Source: CAD feature listing. Evaluate the final solid. Frame: model axes, mm. Round coordinates to 2 decimals unless told otherwise and drop trailing zeros. Loops run counter-clockwise (first coordinate to the right, second up) from the corner with the lowest first, then second, coordinate; pieces in that order, holes last.
Item 1: Section query D-D on z = 0.9. Return loops of the section in (x, y).
Item 2: Ray query, L1, parallel to X at y = 4, z = 1; L2, parallel to X at y = 5, z = 1.2; L3, parallel to Y at x = 31.36, z = 2.05. Return the intervals inside material, ascending.
Item 3: First-contact query: P1, Ø1, axis at y = 30.5, z = 0.5, coming from the -X side; P2, Ø1.5, axis at y = 15.5, z = 1, coming from the +X side; P3, Ø3, axis at x = 23, y = 5, coming from the +Z side; P4, Ø5.5, axis at x = 170, y = 5, coming from the +Z side. Flat tips, straight axial feed; report the tip coordinate or a pass-through.
Item 4: Section query A-A on y = 5. Give the number of separate pieces and of enclosed holes in the cut face, then the cut area to 3 significant figures.
```python
from build123d import *

# Parameters (mm, degrees)
SKETCH1_W                                      = 193
SKETCH1_H                                      = 54
BOSS_EXTRUDE1_DEPTH                            = 3
CHAMFER1_SIZE                                  = 3
CSK_FOR_M3_FLAT_HEAD_MACHINE_SCREW1_AT_2_COUNT = 2
CSK_FOR_M3_FLAT_HEAD_MACHINE_SCREW1_AT_2_PITCH = 73.5
CSK_FOR_M3_FLAT_HEAD_MACHINE_SCREW1_AT_3_COUNT = 2
CSK_FOR_M3_FLAT_HEAD_MACHINE_SCREW1_AT_3_PITCH = 147
SKETCH5_R                                      = 8
CUT_EXTRUDE1_DEPTH                             = 10


with BuildPart() as part:
    # Sketch1 → Boss-Extrude1 (new body)
    with BuildSketch(Plane.XY):
        with Locations((96.5, 27)):
            Rectangle(SKETCH1_W, SKETCH1_H)
    extrude(amount=BOSS_EXTRUDE1_DEPTH)

    # Chamfer1
    chamfer1_edges = [part.edges().sort_by_distance(p)[0] for p in [
        (0, 27, 0),
        (96.5, 54, 0),
        (193, 27, 0),
    ]]
    chamfer(chamfer1_edges, length=CHAMFER1_SIZE - 0.0001)  # a hair under: the kernel refuses the full size

    # Sketch3 → CSK for M3 Flat Head Machine Screw1 (revolve, cut)
    with BuildSketch(Plane(origin=(23, 5, 3), x_dir=(0, -1, 0), z_dir=(1, 0, 0))):
        Polygon((0, 0), (0, 3), (1.7, 3), (1.7, 1.45), (3.15, 0), align=None)
    csk_for_m3_flat_head_machine_screw1 = revolve(axis=Axis((23, 5, 9.35), (0, 0, -1)), mode=Mode.SUBTRACT)

    # CSK for M3 Flat Head Machine Screw1 at 2: CSK for M3 Flat Head Machine Screw1 ×2
    with Locations(*[(i * CSK_FOR_M3_FLAT_HEAD_MACHINE_SCREW1_AT_2_PITCH, 0, 0) for i in range(1, CSK_FOR_M3_FLAT_HEAD_MACHINE_SCREW1_AT_2_COUNT)]):
        add(csk_for_m3_flat_head_machine_screw1, mode=Mode.SUBTRACT)

    # CSK for M3 Flat Head Machine Screw1 at 3: CSK for M3 Flat Head Machine Screw1 ×2
    with Locations(*[(i * CSK_FOR_M3_FLAT_HEAD_MACHINE_SCREW1_AT_3_PITCH, 0, 0) for i in range(1, CSK_FOR_M3_FLAT_HEAD_MACHINE_SCREW1_AT_3_COUNT)]):
        add(csk_for_m3_flat_head_machine_screw1, mode=Mode.SUBTRACT)

    # Sketch5 → Cut-Extrude1 (cut)
    with BuildSketch(Plane.XY.offset(3)):
        with Locations((31.36, 30.75)):
            Circle(SKETCH5_R)
    extrude(amount=-CUT_EXTRUDE1_DEPTH, mode=Mode.SUBTRACT)


solid = part.part
```
Data:
1. outline: (2.1, 0) - (190.9, 0) - (190.9, 51.9) - (2.1, 51.9) - close; hole circle Ø3.4 at (23, 5); hole circle Ø16 at (31.36, 30.75); hole circle Ø3.4 at (96.5, 5); hole circle Ø3.4 at (170, 5)
2. L1: x = 2 to 21.63, 24.37 to 95.13, 97.87 to 168.63, 171.37 to 191
2. L2: x = 1.8 to 21.3, 24.7 to 94.8, 98.2 to 168.3, 171.7 to 191.2
2. L3: y = 0 to 22.75, 38.75 to 53.05
3. P1: stops at x = 2
3. P2: stops at x = 191.75
3. P3: passes through
3. P4: stops at z = 2.6
4. separate pieces: 4
4. enclosed holes: 0
4. area: 533 mm2
